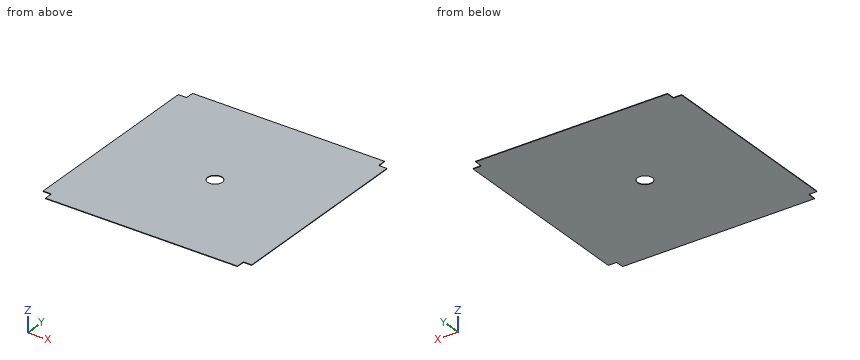
Autodesk Inventor part; units mm, degrees
ref_plane "YZ Plane" through (0, 0, 0) normal (1, 0, 0) x (0, 1, 0)
ref_plane "XZ Plane" through (0, 0, 0) normal (0, 1, 0) x (-1, 0, 0)
ref_plane "XY Plane" through (0, 0, 0) normal (0, 0, 1) x (1, 0, 0)
sketch "Sketch4" plane through (0, 0, 0) normal (0, 0, 1) x (1, 0, 0)
  line L0 (0, 0) -> (500, 0)
  line L1 (500, 0) -> (500, 500)
  line L2 (500, 500) -> (0, 500)
  line L3 (0, 500) -> (0, 0)
  dimension "d9" = 500
  dimension "d10" = 500
extrude "Plate2" add sketch "Sketch4" along normal blind 1.214
sketch "Sketch7" plane through (0, 0, 0) normal (0, 0, 1) x (1, 0, 0)
  line L0 (0, 0) -> (20, 0)
  line L1 (20, 0) -> (20, 20)
  line L2 (20, 20) -> (0, 20)
  line L3 (0, 20) -> (0, 0)
  dimension "d16" = 20
  dimension "d17" = 20
extrude "Cut4" cut sketch "Sketch7" along normal blind 1.214
sketch "Sketch8" plane through (0, 0, 0) normal (0, 0, 1) x (1, 0, 0)
  line L0 (500, 0) -> (500, 500)
  line L1 (500, 0) -> (480, 0)
  line L2 (480, 0) -> (480, 20)
  line L3 (480, 20) -> (500, 20)
  line L4 (500, 20) -> (500, 0)
  line L5 (500, 500) -> (480, 500)
  line L6 (480, 500) -> (480, 480)
  line L7 (480, 480) -> (500, 480)
  line L8 (500, 480) -> (500, 500)
  line L9 (500, 500) -> (0, 500)
  line L10 (0, 500) -> (20, 500)
  line L11 (20, 500) -> (20, 480)
  line L12 (20, 480) -> (0, 480)
  line L13 (0, 480) -> (0, 500)
  point P0 (0, 0)
  dimension "d20" = 20
  dimension "d21" = 20
  dimension "d22" = 20
  dimension "d23" = 20
  dimension "d24" = 20
  dimension "d25" = 20
extrude "Cut5" cut sketch "Sketch8" along normal blind 1.214
sketch "Sketch10" plane through (0, 0, 0) normal (0, 0, 1) x (1, 0, 0)
  line L0 (0, 0) -> (250, 0)
  line L1 (480, 0) -> (20, 0)
  line L2 (0, 0) -> (0, 250)
  line L3 (0, 250) -> (250, 250)
  circle A0 centre (250, 250) radius 17.5
  dimension "d31" = 250
  dimension "d32" = 250
  dimension "d33" = 35
extrude "Cut6" cut sketch "Sketch10" along normal up to next
equation "\"d18\" = Thickness"
equation "\"d26\" = Thickness"
equation "\"d34\" = Thickness"
equation "\"BendRadius\" = Thickness"
equation "\"BendReliefWidth\" = Thickness"
equation "\"BendReliefDepth\" = 0.5 * Thickness"
equation "\"CornerReliefSize\" = 4 * Thickness"
equation "\"MinimumRemnant\" = 2 * Thickness"
equation "\"TransitionRadius\" = BendRadius"
equation "\"JacobiRadiusSize\" = BendRadius"
equation "\"GapSize\" = Thickness"
equation "\"d2\" = BendRadius"
equation "\"d11\" = BendRadius"
properties part number "FrameSheetLaserViewport" material "Steel, Galvanized"
Geometry check sheet. Reference: the model listing, model coordinates, mm. Round coordinates to 2 decimals unless told otherwise and drop trailing zeros. Order: outer loops, then holes, each group sorted by start corner. A loop starts at its lowest first (then second) coordinate and runs counter-clockwise, first axis right, second up. Notation, with made-up numbers: M 85.25,-3 L 140.25,-3 A16 ccw 140.25,6 Z; hole C 16,42.25 d1. An arc over 180 degrees is marked long. Answer in a Markdown table with one row per item. Add a question column.
Item 1: Material ranges on L1, parallel to X at y = 250, z = 0.6; L2, parallel to X at y = 261, z = 0.2, recorded low to high. Write a range as [from, to].
Item 2: Sectioned sample at A-A, the plane x = 250. Enter the section's corners in (y, z), plus the area to 3 significant figures.
Item 3: Depth check by flat-ended pin: pin 1 Ø21 at (x, y) = (250, 250) entering from -Z; pin 2 Ø0.6 at (y, z) = (490.5, 1) entering from +X; pin 3 Ø12 at (x, y) = (112.5, 386) entering from -Z; pin 4 Ø0.6 at (x, z) = (488.5, 0.5) entering from -Y. Enter the tip coordinate at first touch or a pass-through.
Filled in:
| question | item | result |
|---|---|---|
| 1 | L1 | x = [0, 232.5], [267.5, 500] |
| 1 | L2 | x = [0, 236.39], [263.61, 500] |
| 2 | outline | M 0,0 L 232.5,0 L 232.5,1.21 L 0,1.21 Z; M 267.5,0 L 500,0 L 500,1.21 L 267.5,1.21 Z |
| 2 | area | 565 mm² |
| 3 | pin 1 | passes through |
| 3 | pin 2 | stops at x = 480 |
| 3 | pin 3 | stops at z = 0 |
| 3 | pin 4 | stops at y = 20 |
